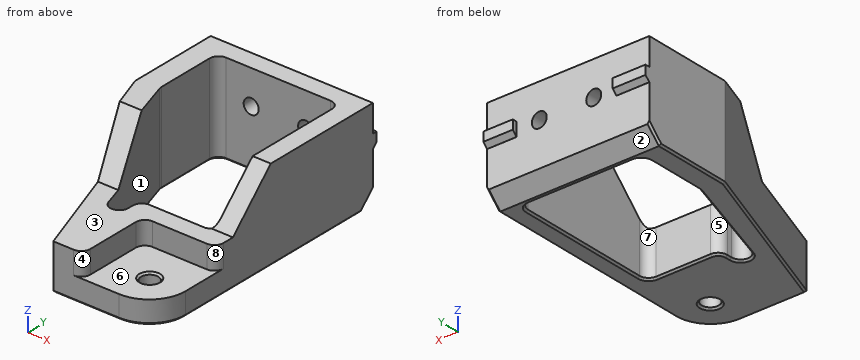
from build123d import *

# Parameters (mm, degrees)
PAD005_DEPTH                               = 20
SKETCH019_W                                = 17
SKETCH019_H                                = 17
POCKET013_DEPTH                            = 15
FILLET004_R                                = 2
SKETCH020_R                                = 1.9
POCKET014_DEPTH                            = 5
FILLET005_R                                = 8
POCKET015_DEPTH                            = 20.001
FILLET006_R                                = 2
POCKET016_DEPTH                            = 36.251
CHAMFER004013007011015006009007001032_SIZE = 3
SKETCH023_R                                = 1.65
POCKET017_DEPTH                            = 5
SKETCH024_W                                = 6.5
SKETCH024_H                                = 3
SKETCH024_W_2                              = 7.25
PAD006_DEPTH                               = 1
CHAMFER004013007011015006009007001033_SIZE = 0.99
CHAMFER004013007011015006009007001034_SIZE = 0.4


with BuildPart() as part:
    # Sketch018 → Pad005 (new body)
    with BuildSketch(Plane.XY):
        Polygon((-28.25, 50), (7.5, 50), (7.5, -7.5), (-15, -7.5), (-28.25, 30), align=None)
    extrude(amount=PAD005_DEPTH)

    # Sketch019 (on Face7 of Pad005) → Pocket013 (cut)
    with BuildSketch(Plane.XY.offset(20)):
        Rectangle(SKETCH019_W, SKETCH019_H)
    extrude(amount=-POCKET013_DEPTH, mode=Mode.SUBTRACT)

    # Fillet004
    fillet004_edges = [part.edges().sort_by_distance(p)[0] for p in [
        (-8.5, -7.5, 12.5),
        (-8.5, 8.5, 12.5),
        (7.5, 8.5, 12.5),
    ]]
    fillet(fillet004_edges, radius=FILLET004_R)

    # Sketch020 (on Face5 of Fillet004) → Pocket014 (cut)
    with BuildSketch(Plane.XY.offset(5)):
        Circle(SKETCH020_R)
    extrude(amount=-POCKET014_DEPTH, mode=Mode.SUBTRACT)

    # Fillet005
    fillet005_edges = [part.edges().sort_by_distance(p)[0] for p in [
        (7.5, -7.5, 2.5),
    ]]
    fillet(fillet005_edges, radius=FILLET005_R)

    # Sketch021 (on DatumPlane) → Pocket015 (cut, through all)
    with BuildSketch(Plane.XY.offset(20)):
        Polygon((-23.5, 31), (-23.5, 46), (3.5, 46), (3.5, 12.5), (-12.5, 12.5), (-12.5, -3.5), align=None)
    extrude(amount=-POCKET015_DEPTH, mode=Mode.SUBTRACT)

    # Fillet006
    fillet006_edges = [part.edges().sort_by_distance(p)[0] for p in [
        (3.5, 12.5, 10),
        (-12.5, 12.5, 10),
        (-12.5, -3.5, 10),
        (-23.5, 31, 10),
        (3.5, 46, 10),
        (-23.5, 46, 10),
    ]]
    fillet(fillet006_edges, radius=FILLET006_R)

    # Sketch022 (on DatumPlane) → Pocket016 (cut, through all)
    with BuildSketch(Plane.YZ.offset(8)):
        Polygon((-8, 10), (13, 10), (23, 20), (-8, 20), align=None)
    extrude(amount=-POCKET016_DEPTH, mode=Mode.SUBTRACT)

    # Chamfer004013007011015006009007001032
    chamfer004013007011015006009007001032_edges = [part.edges().sort_by_distance(p)[0] for p in [
        (-10.375, 50, 0),
    ]]
    chamfer(chamfer004013007011015006009007001032_edges, length=CHAMFER004013007011015006009007001032_SIZE)

    # Sketch023 (on DatumPlane) → Pocket017 (cut)
    with BuildSketch(Plane.XZ.offset(-50)):
        with Locations((-16, 12.5)):
            Circle(SKETCH023_R)
        with Locations((-4, 12.5)):
            Circle(SKETCH023_R)
    extrude(amount=POCKET017_DEPTH, mode=Mode.SUBTRACT)

    # Sketch024 (on DatumPlane) → Pad006 (join)
    with BuildSketch(Plane.XZ.offset(-50)):
        with Locations((4.25, 12.5)):
            Rectangle(SKETCH024_W, SKETCH024_H)
        with Locations((-24.625, 12.5)):
            Rectangle(SKETCH024_W_2, SKETCH024_H)
    extrude(amount=-PAD006_DEPTH)

    # Chamfer004013007011015006009007001033
    chamfer004013007011015006009007001033_edges = [part.edges().sort_by_distance(p)[0] for p in [
        (4.25, 51, 11),
        (-24.625, 51, 11),
    ]]
    chamfer(chamfer004013007011015006009007001033_edges, length=CHAMFER004013007011015006009007001033_SIZE)

    # Chamfer004013007011015006009007001034
    chamfer004013007011015006009007001034_edges = [part.edges().sort_by_distance(p)[0] for p in [
        (7.5, 23.75, 0),
        (5.156854, -5.156854, 0),
        (-7.75, -7.5, 0),
        (-21.625, 11.25, 0),
        (-28.25, 38.5, 0),
        (-28.25, 48.5, 1.5),
        (7.5, 48.5, 1.5),
        (-14.192573, 7.380348, 0),
        (-11.914214, 11.914214, 0),
        (-12.5, 9.92829, 0),
        (-4.5, 12.5, 0),
        (2.914214, 13.085786, 0),
        (3.5, 29.25, 0),
        (2.914214, 45.414214, 0),
        (-10, 46, 0),
        (-22.914214, 45.414214, 0),
        (-23.5, 37.655562, 0),
        (-19.905489, 19.726305, 0),
        (-23.476231, 31.003698, 0),
        (-1.9, 0, 0),
        (-1.9, 0, 5),
    ]]
    chamfer(chamfer004013007011015006009007001034_edges, length=CHAMFER004013007011015006009007001034_SIZE)


solid = part.part
Design review of the part built by this model. Coordinates are the model's own, in mm. Face numbers are marked on the shaded views. A direction names the side the tool comes from. Give positions to 0.01 mm unless a question says otherwise; leave off trailing zeros. Loops run counter-clockwise (first coordinate to the right, second up) from the corner with the lowest first, then second, coordinate; pieces in that order, holes last. Notation, with made-up numbers: (-23.5, 46.25) -> (29.5, 46.25) arc R29 ccw to (29.5, 76.25) -> close; hole circle Ø4 at (10, 45). An arc over 180 degrees is marked (long way). One line per question, with ' | ' between items. Start each with the question number.
(1) For the marked faces 1, 2, 3 and 4, list the 3-axis set-ups (+Z, -Z, +X, -X, +Y, -Y) from which the entire face can be reached by the end or side of a thin tool; tool diameter is ignored.
(2) We need section A-A (x = -4). State the section outline as (y, z) points, and give its area (3 significant figures).
(3) We need section B-B (y = 19). State the section outline as (x, z) points, and give its area (3 significant figures).
(4) Insertion check: P1, Ø2.5, axis at x = -16, z = 12.5, coming from the -Y side; P2, Ø8.5, axis at x = -16.5, z = 7.5, coming from the +Y side; P3, Ø2, axis at x = -3.5, y = 6, coming from the +Z side; P4, Ø0.8, axis at x = 4, y = 50.5, coming from the +Z side. Each pin has a flat end and moves straight along its axis. Give the tip position at first contact, or say it passes through.
(5) We need section C-C (z = 18.75). State the section outline as (x, y) points (3 decimals), and give its area (3 significant figures).
(6) For line 1 (Z direction, x = -4, y = 47); line 2 (X direction, y = 48.75, z = 12.5); line 3 (Z direction, x = -16, y = 48.9), list the stretches that pass through material, from the lowest coordinate up.
(7) Draft analysis for pull direction X (two halves, no side actions). For the marked faces 5, 6, 7 and 8, state which applies: +X half, -X half, draft (parallel to the pull), parting line (faces both ways), or undercut.
The answers:
1) face 1: +Z, -Z | face 2: -Z, +X, -X, +Y | face 3: +Z, +X, -X, -Y | face 4: +Z, +X, -Y
2) outline: (-7.5, 0.4) -> (-7.1, 0) -> (12.1, 0) -> (12.5, 0.4) -> (12.5, 10) -> (8.5, 10) -> (8.5, 5) -> (-7.5, 5) -> close; (46, 0.4) -> (46.4, 0) -> (47, 0) -> (50, 3) -> (50, 10.85) -> (46, 10.85) -> close; (46, 14.15) -> (50, 14.15) -> (50, 20) -> (46, 20) -> close | area: 182 mm^2
3) outline: (-24.36, 0.4) -> (-23.94, 0) -> (-20.09, 0) -> (-19.67, 0.4) -> (-19.67, 16) -> (-24.36, 16) -> close; (3.5, 0.4) -> (3.9, 0) -> (7.1, 0) -> (7.5, 0.4) -> (7.5, 16) -> (3.5, 16) -> close | area: 139 mm^2
4) P1: passes through | P2: stops at y = 50 | P3: stops at z = 5 | P4: stops at z = 14
5) outline: (-28.25, 30) -> (-25.335, 21.75) -> (-20.551, 21.75) -> (-23.405, 30.704) arc R2 cw to (-23.5, 31.311) -> (-23.5, 44) arc R2 cw to (-21.5, 46) -> (1.5, 46) arc R2 cw to (3.5, 44) -> (3.5, 21.75) -> (7.5, 21.75) -> (7.5, 50) -> (-28.25, 50) -> close | area: 359 mm^2
6) line 1: z = 0 to 10.85, 14.15 to 20 | line 2: x = -28.25 to -17.65, -14.35 to -5.65, -2.35 to 7.5 | line 3: z = 1.9 to 10.85, 14.15 to 20
7) face 5: undercut | face 6: draft | face 7: undercut | face 8: +X half
